Autodesk Fusion 360 part; units mm, degrees
sketch "Sketch1" plane through (0, 0, 0) normal (1, 0, 0) x (0, 0, -1)
  circle A0 centre (0, 0) radius 27.5
  dimension "d1" = 55
extrude "Extrude1" add sketch "Sketch1" along normal blind 5
ref_plane "WorkPlane1" through (0, 0, -27.5) normal (0, 0, 1) x (1, 0, 0)
sketch "Sketch2" plane through (0, 0, -27.5) normal (0, 0, 1) x (1, 0, 0)
  line L0 (0, 0) -> (-150, 0)
  line L1 (0, 0) -> (-23, 0)
  line L2 (-150, 0) -> (-110, 0)
  line L3 (0, 0) -> (0, 27.5)
  circle A0 centre (-23, 0) radius 35.8504
  circle A1 centre (-110, 0) radius 40
  line L4 (0, 27.5) -> (0, -27.5)
  arc A2 (-94.2038, 36.7489) -> (-34.165, 34.0675) centre (-60.6369, 114.8402) ccw
  arc A3 (-34.165, -34.0675) -> (-94.2038, -36.7489) centre (-60.6369, -114.8402) ccw
  point P0 (0, -27.5)
  point P1 (0, 27.5)
  dimension "d6" = 150
  dimension "d7" = 23
  dimension "d8" = 40
  dimension "d9" = 27.5
  dimension "d10" = 85
extrude "Extrude2" add sketch "Sketch2" along normal blind 15 contours L0 L1 A0 L4 | L0 L1 L3 A0 L4 | L0 A0 A1 A3 | L0 A0 A1 A2 | L0 L2 A1 | L0 L2 A1
sketch "Sketch3" plane through (0, 0, -27.5) normal (0, 0, -1) x (-1, 0, 0)
  arc A0 (34.165, 34.0675) -> (0, 27.5) centre (23, 0) ccw
  line L0 (0, 27.5) -> (0, 0)
  line L1 (0, 0) -> (0, -27.5)
  arc A1 (0, -27.5) -> (34.165, -34.0675) centre (23, 0) ccw
  arc A2 (94.2038, -36.7489) -> (34.165, -34.0675) centre (60.6369, -114.8402) ccw
  arc A3 (94.2038, -36.7489) -> (94.2038, 36.7489) centre (110, 0) ccw
  arc A4 (34.165, 34.0675) -> (94.2038, 36.7489) centre (60.6369, 114.8402) ccw
  arc A5 (95.1911, -34.4521) -> (95.1911, 34.4521) centre (110, 0) ccw
  arc A6 (33.3864, 31.6918) -> (95.1911, 34.4521) centre (60.6369, 114.8402) ccw
  arc A7 (33.3864, 31.6918) -> (2.5, 26.3059) centre (23, 0) ccw
  line L2 (2.5, 26.3059) -> (2.5, 0)
  line L3 (2.5, 0) -> (2.5, -26.3059)
  arc A8 (2.5, -26.3059) -> (33.3864, -31.6918) centre (23, 0) ccw
  arc A9 (95.1911, -34.4521) -> (33.3864, -31.6918) centre (60.6369, -114.8402) ccw
  dimension "d13" = 2.5
extrude "Extrude3" add sketch "Sketch3" along normal blind 1 contours A5 A6 A7 L2 L3 A8 A9
sketch "Sketch4" plane through (0, 0, -28.5) normal (0, 0, -1) x (-1, 0, 0)
  arc A0 (33.3864, 31.6918) -> (2.5, 26.3059) centre (23, 0) ccw
  line L0 (2.5, 26.3059) -> (2.5, -26.3059)
  arc A1 (2.5, -26.3059) -> (33.3864, -31.6918) centre (23, 0) ccw
  arc A2 (95.1911, -34.4521) -> (33.3864, -31.6918) centre (60.6369, -114.8402) ccw
  arc A3 (95.1911, -34.4521) -> (95.1911, 34.4521) centre (110, 0) ccw
  arc A4 (33.3864, 31.6918) -> (95.1911, 34.4521) centre (60.6369, 114.8402) ccw
  arc A5 (94.2038, -36.7489) -> (94.2038, 36.7489) centre (110, 0) ccw
  arc A6 (34.165, 34.0675) -> (94.2038, 36.7489) centre (60.6369, 114.8402) ccw
  arc A7 (34.165, 34.0675) -> (0, 27.5) centre (23, 0) ccw
  line L1 (0, 27.5) -> (0, -27.5)
  arc A8 (0, -27.5) -> (34.165, -34.0675) centre (23, 0) ccw
  arc A9 (94.2038, -36.7489) -> (34.165, -34.0675) centre (60.6369, -114.8402) ccw
  dimension "d16" = -2.5
extrude "Extrude4" add sketch "Sketch4" along normal blind 5 contours A0 L0 A1 A2 A3 A4 | A5 A6 A7 L1 A8 A9
extrude "Extrude5" add 1 faces at (-110.551, 8.9771, -33.5) along direction (0, 0, -1) blind 6.5 draft -65
sketch "Sketch5" plane through (0, 0, -40) normal (0, 0, -1) x (-1, 0, 0)
  arc A0 (29.8238, 20.8214) -> (99.7085, 23.9425) centre (60.6369, 114.8402) ccw
  arc A1 (29.8238, 20.8214) -> (13.9393, 19.9499) centre (23, 0) ccw
  line L0 (13.9393, 19.9499) -> (13.9393, -19.9499)
  arc A2 (13.9393, -19.9499) -> (29.8238, -20.8214) centre (23, 0) ccw
  arc A3 (99.7085, -23.9425) -> (29.8238, -20.8214) centre (60.6369, -114.8402) ccw
  arc A4 (99.7085, -23.9425) -> (99.7085, 23.9425) centre (110, 0) ccw
  line L1 (150, 0) -> (146, 0)
  circle A5 centre (146, 0) radius 4
  line L2 (146, 4) -> (151, 4)
  line L3 (146, -4) -> (151, -4)
  line L4 (151, 4) -> (151, -4)
  dimension "d21" = 4
  dimension "d22" = 8
  dimension "d23" = 5
extrude "Extrude6" cut sketch "Sketch5" against normal blind 6.5 contours A5 | A5 L2 L3 L4
Read the model definition and answer for the solid it produces. Units are mm, in the model's axes. A direction names the side the tool comes from. Give positions to 0.01 mm unless a question says otherwise; leave off trailing zeros. Write each loop counter-clockwise with the first axis right and the second up, starting at its lowest first coordinate (ties: lowest second). Pieces come first, ordered by that corner, then holes. Notation, with made-up numbers: (-8, 11) -> (12, 11) arc R18 cw to (12, 15) -> close; hole circle Ø4 at (9.5, 5.5). An arc over 180 degrees is marked (long way). Answer as a JSON object with one key per item and string values.
1) A tool of negligible diameter and unlimited length cuts with its end or side. For faces 4 (the cylindrical face through (-64.1, -27.41, -27.99)), 5 (the flat face through (-76, 1, -12.5)), 6 (the flat face through (-69, 30, -28.5)), from which of +Z, -Z, +X, -X, +Y, -Y can it reach the whole face along a straight path? Write none if from no direction.
Findings below:
{"face 4": "-Y", "face 5": "+Z, -X, +Y, -Y", "face 6": "none"}
2) Flat-ended cylindrical pins translate along their axes: pin 1 Ø24 at (x, y) = (-60.5, -3) entering from +Z; pin 2 Ø2 at (y, z) = (-24, 8.5) entering from -X; pin 3 Ø6.5 at (x, y) = (-147, -1.5) entering from -Z. Find the tip coordinate at first contact, or state that the pin passes through.
Findings below:
{"pin 1": "stops at z = -12.5", "pin 2": "stops at x = 0", "pin 3": "stops at z = -35.89"}
3) For a pull along X with two mould halves and no side action, classify faces 1 (the flat face through (0, -21, -22)), 2 (the cylindrical face through (-149.985, -1.107, -20.105)), 3 (the cylindrical face through (-15.983, -35.157, -20.105)) as pulls with the +X half, pulls with the -X half, needs draft (parallel to the pull), parting line crosses it, or undercut.
Findings below:
{"face 1": "pulls with the +X half", "face 2": "parting line crosses it", "face 3": "undercut"}
4) Section C-C on z = 19 is taken. Write down the section's boundary in (x, y), then the cut area to 3 significant figures.
Findings below:
{"outline": "(0, -19.88) -> (5, -19.88) -> (5, 19.88) -> (0, 19.88) -> close", "area": "199 mm^2"}
5) Section B-B on z = 0 is taken. Write down the section's boundary in (x, y), then the cut area to 3 significant figures.
Findings below:
{"outline": "(0, -27.5) -> (5, -27.5) -> (5, 27.5) -> (0, 27.5) -> close", "area": "275 mm^2"}
6) Straight lines are drawn through the part: probe 1 along Y at (x, z) = (-23.5, -23); probe 2 along X at (y, z) = (0.5, 9); probe 3 along Z at (x, y) = (-45, -4.5). For each, find the intervals that lie inside material, in ascending order. Write a range as from..to.
Findings below:
{"probe 1": "y = -35.85..35.85", "probe 2": "x = 0..5", "probe 3": "z = -40..-12.5"}
7) Section A-A on z = -16 is taken. Write down the section's boundary in (x, y) (1 decimal).
Findings below:
{"outline": "(-94.2, -36.7) arc R85 cw to (-34.2, -34.1) arc R35.9 ccw to (0, -27.5) -> (0, -22.4) -> (5, -22.4) -> (5, 22.4) -> (0, 22.4) -> (0, 27.5) arc R35.9 ccw to (-34.2, 34.1) arc R85 cw to (-94.2, 36.7) arc R40 ccw (long way) to start"}
